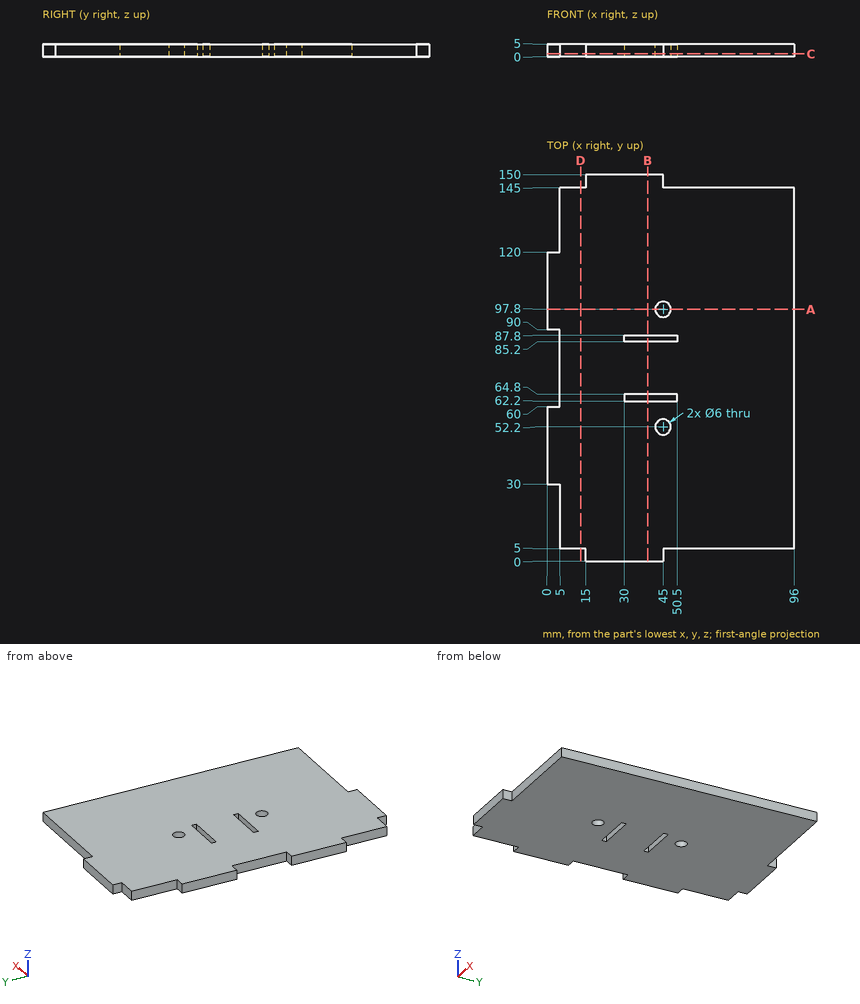
Can you work these out from the drawing? Everything is in mm from the part's minimum corner. Give positions to 0.01 mm unless a question says otherwise; leave off trailing zeros. Loops run counter-clockwise (first coordinate to the right, second up) from the corner with the lowest first, then second, coordinate; pieces in that order, holes last. Notation, with made-up numbers: (21.5, -5.75) - (56.5, -5.75) arc R17 cw to (56.5, 8.25) - close; hole circle Ø9 at (-32, -1). An arc over 180 degrees is marked (long way). Answer as a JSON object with one key per item and string values.
Q1. Imagine slicing it at D-D on x = 13. Write out the boundary of the cut face in (y, z), plus the area to 3 significant figures.
Geometry says:
{"outline": "(5, 0) - (145, 0) - (145, 5) - (5, 5) - close", "area": "700 mm²"}
Q2. Imagine slicing it at C-C on z = 1.15. Give the number of separate pieces and of enclosed holes in the cut face, plus the area to 3 significant figures.
Geometry says:
{"separate pieces": "1", "enclosed holes": "4", "area": "13,200 mm²"}
Q3. If I drill on L1, parallel to Y at x = 49, z = 1.95; L2, parallel to X at y = 98, z = 1.1; L3, parallel to X at y = 126.5, z = 4.15, over which ranges is the centre line in solid material (lowest first)?
Geometry says:
{"L1": "5 to 62.2, 64.8 to 85.2, 87.8 to 145", "L2": "0 to 42.01, 47.99 to 96", "L3": "5 to 96"}
Q4. Imagine slicing it at B-B on x = 39. Write out the boundary of the cut face in (y, z).
Geometry says:
{"outline": "(0, 0) - (62.2, 0) - (62.2, 5) - (0, 5) - close; (64.8, 0) - (85.2, 0) - (85.2, 5) - (64.8, 5) - close; (87.8, 0) - (150, 0) - (150, 5) - (87.8, 5) - close"}
Q5. Imagine slicing it at A-A on y = 97.8. Write out the boundary of the cut face in (x, z), plus the area to 3 significant figures.
Geometry says:
{"outline": "(0, 0) - (42, 0) - (42, 5) - (0, 5) - close; (48, 0) - (96, 0) - (96, 5) - (48, 5) - close", "area": "450 mm²"}
Q6. Will these pins go through, and if not, where does the flat tip stop? P1, Ø2, axis at x = 21.5, y = 110, coming from the -Z side; P2, Ø1.5, axis at y = 23, z = 1.5, coming from the -X side; P3, Ø1.5, axis at x = 3.5, z = 2, coming from the +Y side.
Geometry says:
{"P1": "z = 0", "P2": "x = 5", "P3": "y = 120"}
